Here's how the part is built. I have some questions about the finished solid (model axes, mm). Face numbers are marked on the shaded views. A direction names the side the tool comes from. Round coordinates to 2 decimals unless told otherwise and drop trailing zeros. Write each loop counter-clockwise with the first axis right and the second up, starting at its lowest first coordinate (ties: lowest second). Pieces come first, ordered by that corner, then holes. Notation, with made-up numbers: M -2,-15.5 L 21,-15.5 A17 cw 21,-8.5 Z; hole C 54.5,-28.5 d10. An arc over 180 degrees is marked long. Use a Markdown table: item, result. Add a question column.
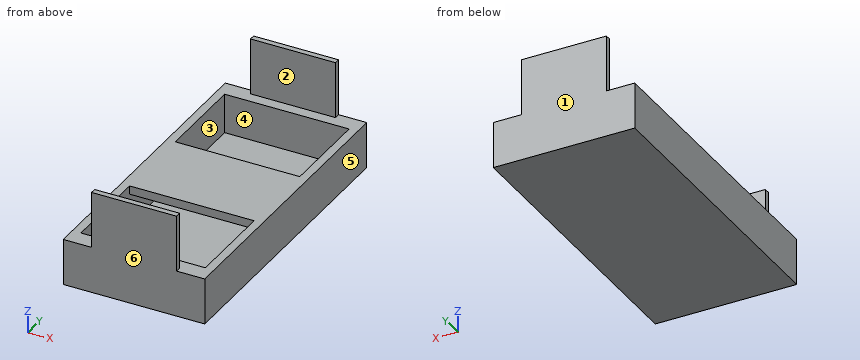
```python
from build123d import *

# Parameters (mm, degrees)
F0_W     = 25
F0_H     = 53.2
F1_DEPTH = 8.2
F2_W     = 15
F2_H     = 1
F3_DEPTH = 10
F4_W     = 22
F4_H     = 47.2
F5_DEPTH = 7
F6_W     = 22
F6_H     = 15
F7_DEPTH = 1.5


with BuildPart() as f1:
    # F0 (on Top) → F1 (new body)
    with BuildSketch(Plane.XY):
        with Locations((12.5, 26.6)):
            Rectangle(F0_W, F0_H)
    extrude(amount=-F1_DEPTH)

    # F2 (on Top) → F3 (join)
    with BuildSketch(Plane.XY):
        with Locations((12.5, 52.7)):
            Rectangle(F2_W, F2_H)
        with Locations((12.5, 0.5)):
            Rectangle(F2_W, F2_H)
    extrude(amount=F3_DEPTH)

    # F4 (on Top) → F5 (cut)
    with BuildSketch(Plane.XY):
        with Locations((12.5, 26.6)):
            Rectangle(F4_W, F4_H)
    extrude(amount=-F5_DEPTH, mode=Mode.SUBTRACT)

    # F6 (on Top) → F7 (join)
    with BuildSketch(Plane.XY):
        with Locations((12.5, 26.5)):
            Rectangle(F6_W, F6_H)
    extrude(amount=-F7_DEPTH)


solid = f1.part
```
Item 1: On a 3-axis mill with a long thin cutter (end or side, diameter ignored), from which of +Z, -Z, +X, -X, +Y, -Y can I reach the whole of each face in a straight line? I mean the marked faces 1, 2 and 3. Say none if no direction works.
Item 2: Imagine slicing it at D-D on z = 5.25. List the corners of the cut face in (x, y) for me, plus the area to 3 significant figures.
Item 3: Imagine slicing it at A-A on x = 19. List the corners of the cut face in (y, z) for me, plus the area to 3 significant figures.
Item 4: Imagine slicing it at C-C on y = 45.5. List the corners of the cut face in (x, z) for me, plus the area to 3 significant figures.
Item 5: If we mould it in two halves opening along X, with no side actions, what happens to the marked faces 4, 5 and 6? For each: +X half, -X half, draft (parallel to the pull), parting line (faces both ways), or undercut.
Item 6: For pin 1 Ø1.1 at (y, z) = (0.5, 3) entering from -X; pin 2 Ø0.8 at (x, z) = (9.5, -0.5) entering from -Y; pin 3 Ø0.8 at (y, z) = (0.5, 3) entering from +X; pin 4 Ø10 at (x, y) = (18.5, 22.5) entering from +Z, each with a flat end and sliding along its axis, tell me the tip position at first contact or that it passes through.
Item 7: Imagine slicing it at B-B on z = -4.5. List the corners of the cut face in (x, y) for me, plus the area to 3 significant figures.
Item 8: I need wall thicknesses on probe 1 along Y at (x, z) = (6, -0.25); probe 2 along X at (y, z) = (34, -6); probe 3 along Z at (x, y) = (14, 32.5). Which ranges of each line are inside material? Lowest first, please. Write a range as from..to.
The answers:
| question | item | result |
|---|---|---|
| 1 | face 1 | +Z, -Z, +X, -X, +Y |
| 1 | face 2 | +Z, +X, -X |
| 1 | face 3 | none |
| 2 | outline | M 5,0 L 20,0 L 20,1 L 5,1 Z; M 5,52.2 L 20,52.2 L 20,53.2 L 5,53.2 Z |
| 2 | area | 30.0 mm² |
| 3 | outline | M 0,-8.2 L 53.2,-8.2 L 53.2,10 L 52.2,10 L 52.2,0 L 50.2,0 L 50.2,-7 L 3,-7 L 3,0 L 1,0 L 1,10 L 0,10 Z; M 19,-1.5 L 34,-1.5 L 34,0 L 19,0 Z |
| 3 | area | 148 mm² |
| 4 | outline | M 0,-8.2 L 25,-8.2 L 25,0 L 23.5,0 L 23.5,-7 L 1.5,-7 L 1.5,0 L 0,0 Z |
| 4 | area | 51.0 mm² |
| 5 | face 4 | undercut |
| 5 | face 5 | +X half |
| 5 | face 6 | draft |
| 6 | pin 1 | x = 5 |
| 6 | pin 2 | y = 0 |
| 6 | pin 3 | x = 20 |
| 6 | pin 4 | z = 0 |
| 7 | outline | M 0,0 L 25,0 L 25,53.2 L 0,53.2 Z; hole M 1.5,3 L 23.5,3 L 23.5,50.2 L 1.5,50.2 Z |
| 7 | area | 292 mm² |
| 8 | probe 1 | 0..3, 19..34, 50.2..53.2 |
| 8 | probe 2 | 0..1.5, 23.5..25 |
| 8 | probe 3 | -8.2..-7, -1.5..0 |
